Build history of the part. All positions in model axes, mm. A direction names the side the tool comes from. Round coordinates to 2 decimals unless told otherwise and drop trailing zeros. Write each loop counter-clockwise with the first axis right and the second up, starting at its lowest first coordinate (ties: lowest second). Pieces come first, ordered by that corner, then holes.
from build123d import *

# Parameters (mm, degrees)
PAD_DEPTH       = 3
SKETCH001_R     = 5.5
SKETCH001_R_2   = 4.5
SKETCH001_W     = 25
SKETCH001_H     = 1.5
SKETCH001_W_2   = 1.5
SKETCH001_H_2   = 15
PAD001_DEPTH    = 1
SKETCH002_R     = 1.5
POCKET_DEPTH    = 264.124048
SKETCH003_R     = 2
POCKET001_DEPTH = 1.5


with BuildPart() as part:
    # Sketch → Pad (new body)
    with BuildSketch(Plane.XY):
        with BuildLine():
            ThreePointArc((-50, 25), (-57.071068, 22.071068), (-60, 15))
            Line((-60, -15), (-60, 15))
            ThreePointArc((-60, -15), (-57.071068, -22.071068), (-50, -25))
            Line((50, -25), (-50, -25))
            ThreePointArc((50, -25), (57.071068, -22.071068), (60, -15))
            Line((60, 15), (60, -15))
            ThreePointArc((60, 15), (57.071068, 22.071068), (50, 25))
            Line((-50, 25), (50, 25))
        make_face()
    extrude(amount=PAD_DEPTH)

    # Sketch001 (on Face10 of Pad) → Pad001 (join)
    with BuildSketch(Plane.XY.offset(3)):
        with Locations((-50, 15)):
            Circle(SKETCH001_R)
        with Locations((-50, 15)):
            Circle(SKETCH001_R_2, mode=Mode.SUBTRACT)
        with Locations((-50, -15)):
            Circle(SKETCH001_R)
        with Locations((-50, -15)):
            Circle(SKETCH001_R_2, mode=Mode.SUBTRACT)
        with Locations((-27.5, 20.75)):
            Rectangle(SKETCH001_W, SKETCH001_H)
        with Locations((-27.5, -20.75)):
            Rectangle(SKETCH001_W, SKETCH001_H)
        with Locations((-55.75, 0)):
            Rectangle(SKETCH001_W_2, SKETCH001_H_2)
    pad001 = extrude(amount=PAD001_DEPTH)

    # Sketch002 (on Face4 of Pad001) → Pocket (cut, through all)
    with BuildSketch(Plane(origin=(0, 0, 0), x_dir=(1, 0, 0), z_dir=(0, 0, -1))):
        with Locations((-50, 15)):
            Circle(SKETCH002_R)
        with Locations((-50, -15)):
            Circle(SKETCH002_R)
    pocket = extrude(amount=-POCKET_DEPTH, mode=Mode.SUBTRACT)

    # Sketch003 (on Face4 of Pocket) → Pocket001 (cut)
    with BuildSketch(Plane(origin=(0, 0, 0), x_dir=(1, 0, 0), z_dir=(0, 0, -1))):
        with Locations((-50, 15)):
            Circle(SKETCH003_R)
        with Locations((-50, -15)):
            Circle(SKETCH003_R)
    pocket001 = extrude(amount=-POCKET001_DEPTH, mode=Mode.SUBTRACT)

    # Mirrored: Pad001, Pocket, Pocket001 across Sketch001 V_Axis
    add(pad001.mirror(Plane(origin=(0, 0, 3), x_dir=(0, 0, 1), z_dir=(1, 0, 0))))
    add(pocket.mirror(Plane(origin=(0, 0, 3), x_dir=(0, 0, 1), z_dir=(1, 0, 0))), mode=Mode.SUBTRACT)
    add(pocket001.mirror(Plane(origin=(0, 0, 3), x_dir=(0, 0, 1), z_dir=(1, 0, 0))), mode=Mode.SUBTRACT)


solid = part.part
1) Slice it at B-B (x = -37). Write the cut outline in (y, z).
Results:
outline: (-25, 0) - (25, 0) - (25, 3) - (21.5, 3) - (21.5, 4) - (20, 4) - (20, 3) - (-20, 3) - (-20, 4) - (-21.5, 4) - (-21.5, 3) - (-25, 3) - close
2) Slice it at D-D (x = 2). Write the cut outline in (y, z), plus the area to 3 significant figures.
Results:
outline: (-25, 0) - (25, 0) - (25, 3) - (-25, 3) - close
area: 150 mm2
3) Which spindle directions (+Z, -Z, +X, -X, +Y, -Y) get a long thin tool onto all of the face, cutting with end or side? Do faces 1 (the cylindrical face through (-51.5, -15.07, 2.24)), 2 (the cylindrical face through (50, 13, 1)), 3 (the flat face through (50, 13, 3)). Say none if no direction does.
Results:
face 1: +Z, -Z
face 2: -Z
face 3: +Z
4) Wall check: L1, parallel to Y at x = -50, z = 2.3; L2, parallel to Y at x = 50, z = 3.5; L3, parallel to X at y = -15, z = 0.75. Give the ranges that are in metal, low to high.
Results:
L1: y = -25 to -16.5, -13.5 to 13.5, 16.5 to 25
L2: y = -20.5 to -19.5, -10.5 to -9.5, 9.5 to 10.5, 19.5 to 20.5
L3: x = -60 to -52, -48 to 48, 52 to 60
5) Slice it at C-C (z = 0.65). Write the cut outline in (x, y), plus the area to 3 significant figures.
Results:
outline: (-60, -15) arc R10 ccw to (-50, -25) - (50, -25) arc R10 ccw to (60, -15) - (60, 15) arc R10 ccw to (50, 25) - (-50, 25) arc R10 ccw to (-60, 15) - close; hole circle Ø4 at (-50, -15); hole circle Ø4 at (-50, 15); hole circle Ø4 at (50, -15); hole circle Ø4 at (50, 15)
area: 5,860 mm2
6) Slice it at A-A (y = -2.5). Write the cut outline in (x, z).
Results:
outline: (-60, 0) - (60, 0) - (60, 3) - (56.5, 3) - (56.5, 4) - (55, 4) - (55, 3) - (-55, 3) - (-55, 4) - (-56.5, 4) - (-56.5, 3) - (-60, 3) - close
7) Pin check, flat tips, straight feed: pin 1 Ø1.1 at (x, z) = (-26.5, 3.5) entering from -Y; pin 2 Ø1.2 at (x, y) = (50, -15.5) entering from -Z; pin 3 Ø0.8 at (x, z) = (30.5, 3.5) entering from +Y; pin 4 Ø0.8 at (y, z) = (-20.5, 3.5) entering from -X. Stop position of each tip, or through.
Results:
pin 1: stops at y = -25
pin 2: passes through
pin 3: stops at y = 21.5
pin 4: stops at x = -52.06
